from build123d import *

# Parameters (mm, degrees)
BOSS_EXTRUDE1_DEPTH     = 3.175
FILLET1_R               = 12.7
F_1_4_CLEARANCE_HOLE1_D = 6.7564
F_1_4_CLEARANCE_HOLE3_D = 6.7564
F_1_4_CLEARANCE_HOLE4_D = 6.7564
SKETCH11_R              = 3.3782
BOSS_EXTRUDE2_DEPTH     = 6.35
FILLET2_R               = 12.7
SKETCH12_R              = 3.3782
CUT_EXTRUDE1_DEPTH      = 302.94233307


with BuildPart() as part:
    # Sketch1 → Boss-Extrude1 (new, symmetric)
    with BuildSketch(Plane.XY):
        Polygon((-88.9, 0), (-114.3, 0), (-114.3, 62.644214517), (-41.726805286, 123.540355435), (-12.7, 147.896737045), (-12.7, 279.4), (12.7, 279.4), (12.7, 147.896737045), (41.726805286, 123.540355435), (114.3, 62.644214517), (114.3, 0), (88.9, 0), (88.9, 50.8), (25.4, 104.08282658), (0, 125.395957212), (-25.4, 104.08282658), (-88.9, 50.8), align=None)
    extrude(amount=BOSS_EXTRUDE1_DEPTH, both=True)

    # Fillet1
    fillet1_edges = [part.edges().sort_by_distance(p)[0] for p in [
        (-114.3, 62.644214517, 0),
        (-12.7, 147.896737045, 0),
        (12.7, 147.896737045, 0),
        (114.3, 62.644214517, 0),
        (88.9, 50.8, 0),
        (0, 125.395957212, 0),
        (-88.9, 50.8, 0),
    ]]
    fillet(fillet1_edges, radius=FILLET1_R)

    # 1/4 Clearance Hole1 (through all)
    with Locations(Plane.XY.offset(3.175)):
        with Locations((101.6, 34.925), (-101.6, 9.525), (-101.6, 34.925), (101.6, 9.525)):
            Hole(F_1_4_CLEARANCE_HOLE1_D / 2)

    # 1/4 Clearance Hole3 (through all)
    with Locations(Plane(origin=(0, 0, -3.175), x_dir=(-1, 0, 0), z_dir=(0, 0, -1))):
        with Locations((0, 134.62)):
            Hole(F_1_4_CLEARANCE_HOLE3_D / 2)

    # 1/4 Clearance Hole4 (through all)
    with Locations(Plane.XY.offset(3.175)):
        with Locations((0, 217.046839415)):
            Hole(F_1_4_CLEARANCE_HOLE4_D / 2)

    # Sketch11 → Boss-Extrude2 (add)
    with BuildSketch(Plane.XY.offset(3.175)):
        with BuildLine():
            Line((-43.303160585, 279.4), (43.303160585, 279.4))
            Line((43.303160585, 279.4), (43.303160585, 274.196839415))
            ThreePointArc((43.303160585, 274.196839415), (42.805221287, 271.975629672), (41.406708366, 270.179556768))
            Line((41.406708366, 270.179556768), (2.60825781, 238.24375032))
            ThreePointArc((2.60825781, 238.24375032), (0, 239.475039415), (-2.60825781, 238.24375032))
            Line((-2.60825781, 238.24375032), (-41.406708366, 270.179556768))
            ThreePointArc((-41.406708366, 270.179556768), (-42.805221287, 271.975629672), (-43.303160585, 274.196839415))
            Line((-43.303160585, 274.196839415), (-43.303160585, 279.4))
        make_face()
        with Locations((-38.1, 274.196839415)):
            Circle(SKETCH11_R, mode=Mode.SUBTRACT)
        with Locations((38.1, 274.196839415)):
            Circle(SKETCH11_R, mode=Mode.SUBTRACT)
    extrude(amount=-BOSS_EXTRUDE2_DEPTH)

    # Fillet2
    fillet2_edges = [part.edges().sort_by_distance(p)[0] for p in [
        (12.7, 246.550471869, 0),
        (-12.7, 246.550471869, 0),
    ]]
    fillet(fillet2_edges, radius=FILLET2_R)

    # Sketch12 → Cut-Extrude1 (cut, through all)
    with BuildSketch(Plane.XY.offset(3.175)):
        with Locations((0, 236.096839415)):
            Circle(SKETCH12_R)
    extrude(amount=-CUT_EXTRUDE1_DEPTH, mode=Mode.SUBTRACT)


solid = part.part
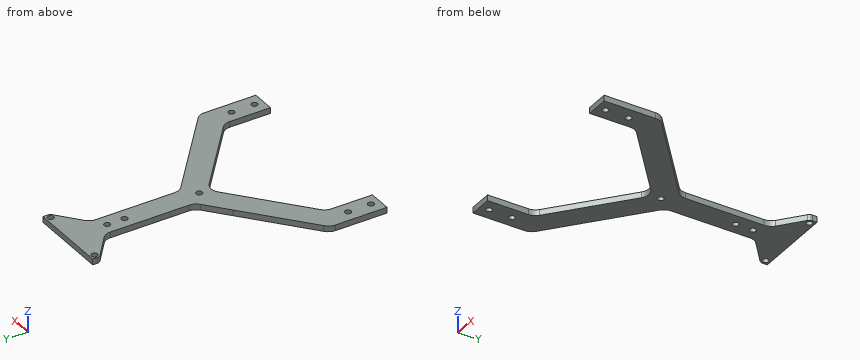
The listing builds one solid part. Answer for the finished solid, in the listing's coordinates (mm). Round coordinates to 2 decimals unless told otherwise and drop trailing zeros. Order: outer loops, then holes, each group sorted by start corner. A loop starts at its lowest first (then second) coordinate and runs counter-clockwise, first axis right, second up. Notation, with made-up numbers: (65.25, -12) - (114.25, -12) arc R19 ccw to (114.25, 25) - close; hole circle Ø9 at (-36, 65). An arc over 180 degrees is marked (long way). Write item = value, one per line. Start each with the question number.
1) Section B-B, the plane x = -38.1 is taken. Write down the section's boundary in (y, z) (3 decimals).
2) Section C-C, the plane y = 134.62 is taken. Write down the section's boundary in (x, z) (3 decimals).
3) Section D-D, the plane z = 2 is taken. Count the separate pieces of the cut face and the enclosed holes in it, plus the area to 3 significant figures.
4) Straight lines are drawn through the part: L1, parallel to Y at x = 0, z = -0.5; L2, parallel to X at y = 31.5, z = 2.5; L3, parallel to X at y = 12.5, z = -2.25. For each, find the intervals that lie inside material, in ascending order.
5) Section A-A, the plane x = 0 is taken. Write down the section's boundary in (y, z) (3 decimals).
6) Given pin 1 (11 mm diameter, centred on x = -101.6, y = 9.525, fed in from -Z) (3 decimals); pin 2 (2.5 mm diameter, centred on y = 275.5, z = 0, fed in from +X); pin 3 (1 mm diameter, centred on y = 242.5, z = 1.5, fed in from +X); pin 4 (1.9 mm diameter, centred on y = 198, z = -0.5, fed in from -X), each flat-ended and moving along its own axis, determine where each tip first touches the part or whether it passes through.
Results list:
q1.outline = (93.426, -3.175) - (126.584, -3.175) - (126.584, 3.175) - (93.426, 3.175) - close; (267.458, -3.175) - (270.819, -3.175) - (270.819, 3.175) - (267.458, 3.175) - close; (277.575, -3.175) - (279.4, -3.175) - (279.4, 3.175) - (277.575, 3.175) - close
q2.outline = (-28.523, -3.175) - (-3.378, -3.175) - (-3.378, 3.175) - (-28.523, 3.175) - close; (3.378, -3.175) - (28.523, -3.175) - (28.523, 3.175) - (3.378, 3.175) - close
q3.separate_pieces = 1
q3.enclosed_holes = 9
q3.area = 13,800 mm^2
q4.L1 = 121.52 to 131.24, 138 to 213.67, 220.43 to 232.72, 239.48 to 279.4
q4.L2 = -114.3 to -88.9, 88.9 to 114.3
q4.L3 = -114.3 to -103.2, -100 to -88.9, 88.9 to 100, 103.2 to 114.3
q5.outline = (121.517, -3.175) - (131.242, -3.175) - (131.242, 3.175) - (121.517, 3.175) - close; (137.998, -3.175) - (213.669, -3.175) - (213.669, 3.175) - (137.998, 3.175) - close; (220.425, -3.175) - (232.719, -3.175) - (232.719, 3.175) - (220.425, 3.175) - close; (239.475, -3.175) - (279.4, -3.175) - (279.4, 3.175) - (239.475, 3.175) - close
q6.pin_1 = -3.175
q6.pin_2 = 43.3
q6.pin_3 = 12.94
q6.pin_4 = -12.7
